CAD build for the part. Positions are in the model's coordinates, mm. A direction names the side the tool comes from. Round coordinates to 2 decimals unless told otherwise and drop trailing zeros. Write each loop counter-clockwise with the first axis right and the second up, starting at its lowest first coordinate (ties: lowest second). Pieces come first, ordered by that corner, then holes. Notation, with made-up numbers: (44.5, 36.5) -> (56.5, 36.5) arc R20 cw to (56.5, 55.5) -> close; hole circle Ø3 at (-7, -11.75). An arc over 180 degrees is marked (long way). Put each result on its own line as item: value. Start each with the question number.
1. 3-axis set-ups, long thin cutter, end or side, ignore diameter. For faces 1 (the flat face through (170, -79, 0)), 2 (the flat face through (369, 0, 5)), 3 (the flat face through (170, -79, -5)): which of +Z, -Z, +X, -X, +Y, -Y reach the whole face in a straight line?
2. Pull direction Y, two halves, no side cores. Call faces 4 (the flat face through (369.736, -81.12, 2.334)), 5 (the flat face through (175, -160, -23)), 6 (the flat face through (369, -160, 5)): pulls with the +Y half, pulls with the -Y half, needs draft (parallel to the pull), parting line crosses it, or undercut.
3. Saw through at C-C on y = -141. List the corners of the cut face in (x, z).
4. Saw through at B-B on x = 70.5. List the corners of the cut face in (y, z).
5. Saw through at A-A on z = -24.5. List the corners of the cut face in (x, y), and give its area (3 significant figures).
6. Flat gauge pins, fed straight in: P1, Ø4.5, axis at y = -161, z = -14.5, coming from the +X side; P2, Ø9.5, axis at x = 363, z = 7, coming from the +Y side; P3, Ø4, axis at x = 160, y = -138, coming from the +Z side. Where does each tip first touch, or does it go through?
7. Drill centre lines: line 1 (Y direction, x = 325, z = -17.5); line 2 (Z direction, x = 265, y = -143.5); line 3 (Z direction, x = 361, y = -84). Where is each one in solid material? Low to high. Write a range as from..to.
from build123d import *

# Parameters (mm, degrees)
SKETCH1_W                      = 345
SKETCH1_H                      = 160
BASE_FLANGE1_DEPTH             = 5
EDGE_FLANGE1_STRIP_CUT_DEPTH   = 160
EDGE_FLANGE1_DEPTH             = 160
EDGE_FLANGE2_STRIP_W           = 21.4732
EDGE_FLANGE2_STRIP_H           = 5
EDGE_FLANGE2_STRIP_CUT_DEPTH   = 344.889914392
EDGE_FLANGE2_STRIP_2_W         = 21.4732
EDGE_FLANGE2_STRIP_2_H         = 5
EDGE_FLANGE2_STRIP_CUT_2_DEPTH = 344.889914392
EDGE_FLANGE2_DEPTH             = 344.889914392
EDGE_FLANGE2_BEND_DEPTH        = 344.889914392


# Sheet-metal steps are written as plain solids
with BuildPart() as part:
    # Sketch1 → Base-Flange1 (new body)
    with BuildSketch(Plane.XY):
        with Locations((172.5, -80)):
            Rectangle(SKETCH1_W, SKETCH1_H)
    extrude(amount=-BASE_FLANGE1_DEPTH)

    # Edge-Flange1 strip (across the edge) → Edge-Flange1 strip cut (cut)
    with BuildSketch(Plane(origin=(345, -160, 0), x_dir=(-0.29237170472273066, 0, 0.9563047559630373), z_dir=(0, 1, 0))):
        Polygon((-11.027493953, 18.967789372), (-4.749337863, -1.567133914), (0.032185917, -0.10527539), (-6.245970173, 20.429647896), align=None)
    extrude(amount=EDGE_FLANGE1_STRIP_CUT_DEPTH, mode=Mode.SUBTRACT)

    # Edge-Flange1 section (across the edge) → Edge-Flange1 (add)
    with BuildSketch(Plane(origin=(345, -160, 0), x_dir=(-0.29237170472273066, 0, 0.9563047559630373), z_dir=(0, 1, 0))):
        with BuildLine():
            Line((-5, 0.110085608), (-5, 49.252744993))
            Line((-5, 49.252744993), (0, 49.252744993))
            Line((0, 49.252744993), (0, 0.110085608))
            ThreePointArc((0, 0.110085608), (0.008090915, 0.001209195), (0.032185917, -0.10527539))
            Line((0.032185917, -0.10527539), (-4.749337863, -1.567133914))
            ThreePointArc((-4.749337863, -1.567133914), (-4.936988402, -0.73783786), (-5, 0.110085608))
        make_face()
    extrude(amount=EDGE_FLANGE1_DEPTH)

    # Edge-Flange2 strip (across the edge) → Edge-Flange2 strip cut (cut)
    with BuildSketch(Plane(origin=(344.889914392, -160, -5), x_dir=(0, 1, 0), z_dir=(-1, 0, 0))):
        with Locations((-10, -2.5)):
            Rectangle(EDGE_FLANGE2_STRIP_W, EDGE_FLANGE2_STRIP_H)
    extrude(amount=EDGE_FLANGE2_STRIP_CUT_DEPTH, mode=Mode.SUBTRACT)

    # Edge-Flange2 strip 2 (across the edge) → Edge-Flange2 strip cut 2 (cut)
    with BuildSketch(Plane(origin=(0, 0, -5), x_dir=(0, -1, 0), z_dir=(1, 0, 0))):
        with Locations((-10, -2.5)):
            Rectangle(EDGE_FLANGE2_STRIP_2_W, EDGE_FLANGE2_STRIP_2_H)
    extrude(amount=EDGE_FLANGE2_STRIP_CUT_2_DEPTH, mode=Mode.SUBTRACT)

    # Edge-Flange2 section (across the edge) → Edge-Flange2 (add)
    with BuildSketch(Plane(origin=(344.889914392, -160, -5), x_dir=(0, 1, 0), z_dir=(-1, 0, 0))):
        with BuildLine():
            Line((-5, 0.7366), (-5, 35))
            Line((-5, 35), (0, 35))
            Line((0, 35), (0, 0.7366))
            ThreePointArc((0, 0.7366), (0.215745145, 0.215745145), (0.7366, 0))
            Line((0.7366, 0), (0.7366, -5))
            ThreePointArc((0.7366, -5), (-3.319788761, -3.319788761), (-5, 0.7366))
        make_face()
    extrude(amount=EDGE_FLANGE2_DEPTH)

    # Edge-Flange2 section 2 (across the edge) → Edge-Flange2 bend (add)
    with BuildSketch(Plane(origin=(0, 0, -5), x_dir=(0, -1, 0), z_dir=(1, 0, 0))):
        with BuildLine():
            Line((-5, 0.7366), (-5, 35))
            Line((-5, 35), (0, 35))
            Line((0, 35), (0, 0.7366))
            ThreePointArc((0, 0.7366), (0.215745145, 0.215745145), (0.7366, 0))
            Line((0.7366, 0), (0.7366, -5))
            ThreePointArc((0.7366, -5), (-3.319788761, -3.319788761), (-5, 0.7366))
        make_face()
    extrude(amount=EDGE_FLANGE2_BEND_DEPTH)


solid = part.part
Return value:
1. face 1: +Z, -X, +Y, -Y
1. face 2: +Z, -Z, +X, +Y
1. face 3: -Z, +X, -X
2. face 4: needs draft
2. face 5: undercut
2. face 6: pulls with the -Y half
3. outline: (0, -5) -> (344.89, -5) arc R5.74 ccw to (346.57, -4.75) -> (393.56, 9.62) -> (392.1, 14.4) -> (345.11, 0.03) arc R0.74 cw to (344.89, 0) -> (0, 0) -> close
4. outline: (-165, -40) -> (-160, -40) -> (-160, -5.74) arc R0.74 cw to (-159.26, -5) -> (-0.74, -5) arc R0.74 cw to (0, -5.74) -> (0, -40) -> (5, -40) -> (5, -5.74) arc R5.74 ccw to (-0.74, 0) -> (-159.26, 0) arc R5.74 ccw to (-165, -5.74) -> close
5. outline: (0, -165) -> (344.89, -165) -> (344.89, -160) -> (0, -160) -> close; (0, 0) -> (344.89, 0) -> (344.89, 5) -> (0, 5) -> close
5. area: 3,450 mm^2
6. P1: stops at x = 344.89
6. P2: stops at y = 0
6. P3: stops at z = 0
7. line 1: y = -165..-160, 0..5
7. line 2: z = -5..0
7. line 3: z = -0.34..4.89
